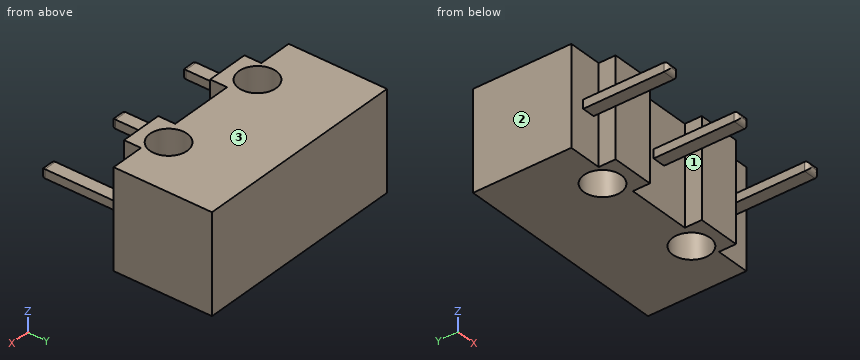
```python
from build123d import *

# Parameters (mm, degrees)
SKETCH_1_W          = 12.8
SKETCH_1_H          = 5.8
EXTRUDE_1_DEPTH     = 5.8
SKETCH_2_W          = 0.76
SKETCH_2_H          = 0.52
EXTRUDE_2_DEPTH     = 5
FILLET_3_R          = 0.25
SKETCH_4_W          = 2.5
SKETCH_4_H          = 5.8
EXTRUDE_3_DEPTH     = 1
SKETCH_3_R          = 1.1
CUT_EXTRUDE_1_DEPTH = 11.403845443


with BuildPart() as part:
    # 草图1 → 凸台-拉伸1 (new body)
    with BuildSketch(Plane(origin=(0, 0, 0), x_dir=(1, 0, 0), z_dir=(0, 1, 0))):
        Rectangle(SKETCH_1_W, SKETCH_1_H)
    extrude(amount=EXTRUDE_1_DEPTH)

    # 草图2 → 凸台-拉伸2 (add)
    with BuildSketch(Plane.XZ):
        Rectangle(SKETCH_2_W, SKETCH_2_H)
        with Locations((5.15, 0)):
            Rectangle(SKETCH_2_W, SKETCH_2_H)
        with Locations((-5.15, 0)):
            Rectangle(SKETCH_2_W, SKETCH_2_H)
    extrude(amount=EXTRUDE_2_DEPTH)

    # 圆角3
    fillet_3_edges = [part.edges().sort_by_distance(p)[0] for p in [
        (0.38, -5, 0),
        (0, -5, 0.26),
        (-0.38, -5, 0),
        (0, -5, -0.26),
        (5.15, -5, 0.26),
        (4.77, -5, 0),
        (5.15, -5, -0.26),
        (5.53, -5, 0),
        (-4.77, -5, 0),
        (-5.15, -5, 0.26),
        (-5.53, -5, 0),
        (-5.15, -5, -0.26),
    ]]
    fillet(fillet_3_edges, radius=FILLET_3_R)

    # 草图4 → 凸台-拉伸3 (add)
    with BuildSketch(Plane.XZ):
        with Locations((-3.15, 0)):
            Rectangle(SKETCH_4_W, SKETCH_4_H)
        with Locations((3.15, 0)):
            Rectangle(SKETCH_4_W, SKETCH_4_H)
    extrude(amount=EXTRUDE_3_DEPTH)

    # 草图3 → 切除-拉伸1 (cut, through all)
    with BuildSketch(Plane.XY.offset(2.9)):
        with Locations((-3.25, 0.7)):
            Circle(SKETCH_3_R)
        with Locations(Location((3.25, 0.7, 0), (0, 0, 180))):
            Circle(SKETCH_3_R)
    extrude(amount=-CUT_EXTRUDE_1_DEPTH, mode=Mode.SUBTRACT)


solid = part.part
```
Check sheet for the modelled part. Datum: model origin and axes. Units: mm. Face numbers are marked on the shaded views. Round coordinates to 2 decimals unless told otherwise and drop trailing zeros. Order: outer loops, then holes, each group sorted by start corner. A loop starts at its lowest first (then second) coordinate and runs counter-clockwise, first axis right, second up.
1) Mould release check, pull along X, two halves, no side actions. Record for the marked faces 1, 2 and 3: +X half, -X half, draft (parallel to the pull), parting line (faces both ways), or undercut.
2) Section check B-B (x = 3.25). Record the boundary of the cut face in (y, z), and give its area (3 significant figures).
3) Section check A-A (y = -2). Record the boundary of the cut face in (x, z).
4) Section check D-D (y = 0.7). Record the boundary of the cut face in (x, z), and give its area (3 significant figures).
5) Section check C-C (z = 1.65). Record the boundary of the cut face in (x, y).
6) Scan lines: line 1 (X direction, y = -3.75, z = 0.2); line 2 (Y direction, x = 3.25, z = 1.55); line 3 (X direction, y = -0.75, z = -0.7). Record each from-to range of solid material in increasing order.
7) Go/stop test with flat-tipped pins: pin 1 Ø1.3 at (x, z) = (-3.5, 0.5) entering from -Y; pin 2 Ø0.6 at (y, z) = (-2, 0) entering from +X; pin 3 Ø0.6 at (x, y) = (5, -2) entering from -Z. Record where each tip stops, or that it passes through.
Result:
1. face 1: undercut
1. face 2: -X half
1. face 3: draft
2. outline: (-1, -2.9) - (-0.4, -2.9) - (-0.4, 2.9) - (-1, 2.9) - close; (1.8, -2.9) - (5.8, -2.9) - (5.8, 2.9) - (1.8, 2.9) - close
2. area: 26.7 mm2
3. outline: (-5.53, -0.26) - (-4.77, -0.26) - (-4.77, 0.26) - (-5.53, 0.26) - close; (-0.38, -0.26) - (0.38, -0.26) - (0.38, 0.26) - (-0.38, 0.26) - close; (4.77, -0.26) - (5.53, -0.26) - (5.53, 0.26) - (4.77, 0.26) - close
4. outline: (-6.4, -2.9) - (-4.35, -2.9) - (-4.35, 2.9) - (-6.4, 2.9) - close; (-2.15, -2.9) - (2.15, -2.9) - (2.15, 2.9) - (-2.15, 2.9) - close; (4.35, -2.9) - (6.4, -2.9) - (6.4, 2.9) - (4.35, 2.9) - close
4. area: 48.7 mm2
5. outline: (-6.4, 0) - (-4.4, 0) - (-4.4, -1) - (-1.9, -1) - (-1.9, 0) - (1.9, 0) - (1.9, -1) - (4.4, -1) - (4.4, 0) - (6.4, 0) - (6.4, 5.8) - (-6.4, 5.8) - close; hole circle Ø2.2 at (-3.25, 0.7); hole circle Ø2.2 at (3.25, 0.7)
6. line 1: x = -5.53 to -4.77, -0.38 to 0.38, 4.77 to 5.53
6. line 2: y = -1 to -0.4, 1.8 to 5.8
6. line 3: x = -4.4 to -1.9, 1.9 to 4.4
7. pin 1: stops at y = -1
7. pin 2: stops at x = 5.53
7. pin 3: stops at z = -0.26
